For this review, take the finished solid that the model builds, in its own axes (mm). Coordinates: 2 decimals unless noted, no trailing zeros. Loops run counter-clockwise (first coordinate to the right, second up) from the corner with the lowest first, then second, coordinate; pieces in that order, holes last. Notation, with made-up numbers: (-16, 57.25) -> (20, 57.25) arc R32 ccw to (20, 84.25) -> close; hole circle Ø7 at (37.25, -15). An arc over 180 degrees is marked (long way). Answer in a Markdown table with one row per item.
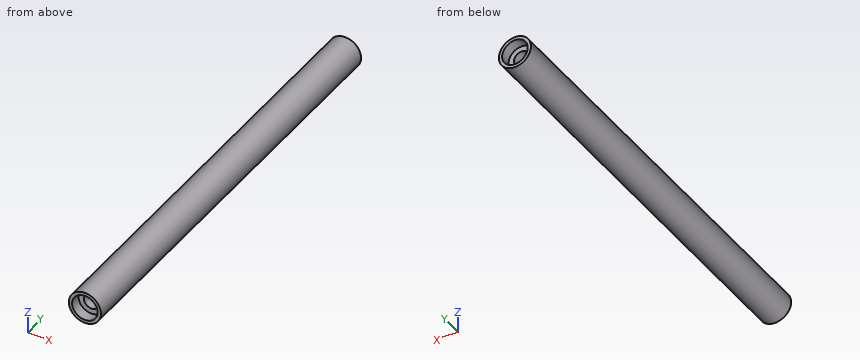
from build123d import *

# Parameters (mm, degrees)
SKETCH_1_R          = 7.5
EXTRUDE_1_DEPTH     = 200
SKETCH_2_R          = 3.5
CUT_EXTRUDE_1_DEPTH = 201
SKETCH_4_R          = 6
CUT_EXTRUDE_3_DEPTH = 5
SKETCH_7_R          = 6
CUT_EXTRUDE_4_DEPTH = 5


with BuildPart() as part:
    # Эскиз1 → Бобышка-Вытянуть1 (new body)
    with BuildSketch(Plane(origin=(0, 0, 0), x_dir=(1, 0, 0), z_dir=(0, 1, 0))):
        Circle(SKETCH_1_R)
    extrude(amount=EXTRUDE_1_DEPTH)

    # Эскиз2 → Вырез-Вытянуть1 (cut, through all)
    with BuildSketch(Plane(origin=(0, 200, 0), x_dir=(1, 0, 0), z_dir=(0, 1, 0))):
        Circle(SKETCH_2_R)
    extrude(amount=-CUT_EXTRUDE_1_DEPTH, mode=Mode.SUBTRACT)

    # Эскиз4 → Вырез-Вытянуть3 (cut)
    with BuildSketch(Plane(origin=(0, 200, 0), x_dir=(1, 0, 0), z_dir=(0, 1, 0))):
        Circle(SKETCH_4_R)
    extrude(amount=-CUT_EXTRUDE_3_DEPTH, mode=Mode.SUBTRACT)

    # Эскиз7 → Вырез-Вытянуть4 (cut)
    with BuildSketch(Plane.XZ):
        Circle(SKETCH_7_R)
    extrude(amount=-CUT_EXTRUDE_4_DEPTH, mode=Mode.SUBTRACT)


solid = part.part
Item 1: Take a section at C-C, the plane y = 162.5. State the section outline as (x, z) points, and give its area (3 significant figures).
Worked answers:
| item | result |
|---|---|
| outline | circle Ø15 at (0, 0); hole circle Ø7 at (0, 0) |
| area | 138 mm² |
Item 2: Take a section at B-B, the plane z = 0. State the section outline as (x, y) points, and give its area (3 significant figures).
Worked answers:
| item | result |
|---|---|
| outline | (-7.5, 0) -> (-6, 0) -> (-6, 5) -> (-3.5, 5) -> (-3.5, 195) -> (-6, 195) -> (-6, 200) -> (-7.5, 200) -> close; (3.5, 5) -> (6, 5) -> (6, 0) -> (7.5, 0) -> (7.5, 200) -> (6, 200) -> (6, 195) -> (3.5, 195) -> close |
| area | 1,550 mm² |
Item 3: For L1, parallel to X at y = 107, z = 0; L2, parallel to Z at x = 0, y = 196.85, list the stretches that pass through material, from the lowest coordinate up.
Worked answers:
| item | result |
|---|---|
| L1 | -7.5 to -3.5, 3.5 to 7.5 |
| L2 | -7.5 to -6, 6 to 7.5 |
Item 4: Take a section at A-A, the plane x = 0. State the section outline as (y, z) points.
Worked answers:
| item | result |
|---|---|
| outline | (0, -7.5) -> (200, -7.5) -> (200, -6) -> (195, -6) -> (195, -3.5) -> (5, -3.5) -> (5, -6) -> (0, -6) -> close; (0, 6) -> (5, 6) -> (5, 3.5) -> (195, 3.5) -> (195, 6) -> (200, 6) -> (200, 7.5) -> (0, 7.5) -> close |
Item 5: Insertion check: pin 1 (1.5 mm diameter, centred on y = 123, z = -4, fed in from +X); pin 2 (4 mm diameter, centred on x = -1, z = 5, fed in from -Y); pin 3 (3 mm diameter, centred on x = -3, y = 93, fed in from +Z); pin 4 (3 mm diameter, centred on x = 3, y = 113.5, fed in from -Z). Each pin has a flat end and moves straight along its axis. Give the tip position at first contact, or say it passes through.
Worked answers:
| item | result |
|---|---|
| pin 1 | x = 6.76 |
| pin 2 | y = 0 |
| pin 3 | z = 7.35 |
| pin 4 | z = -7.35 |
